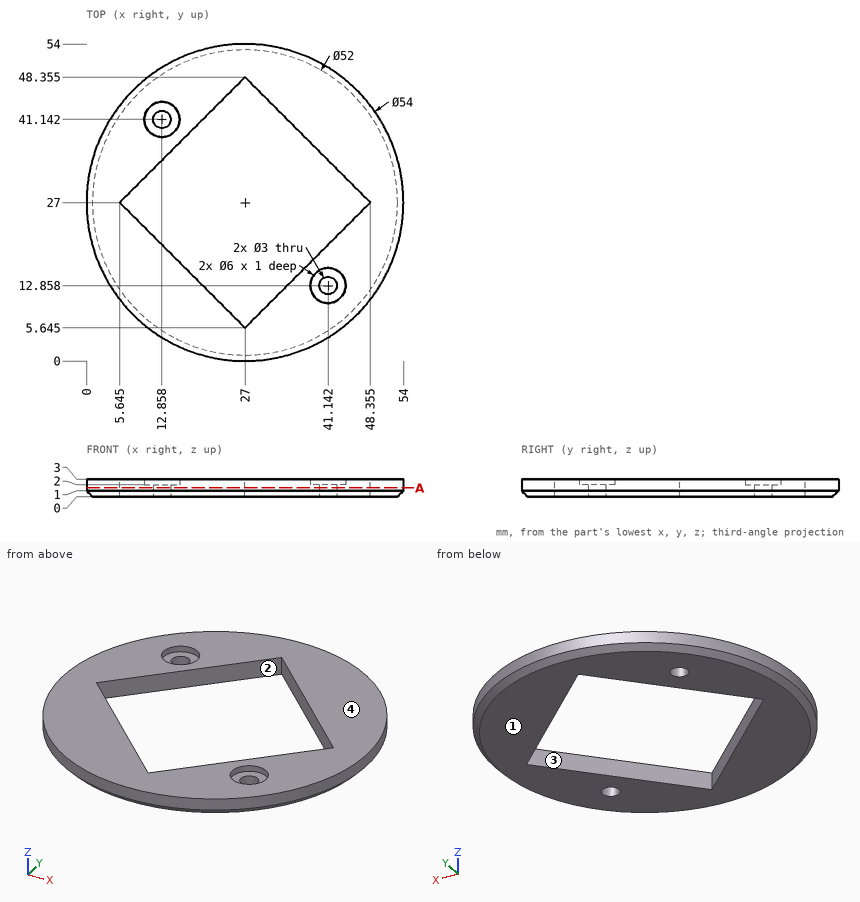
Input: dimensioned drawing with shaded views. Units: mm. Origin: part minimum x, y, z. A direction names the side the tool comes from. Round coordinates to 2 decimals unless told otherwise and drop trailing zeros. Loops run counter-clockwise (first coordinate to the right, second up) from the corner with the lowest first, then second, coordinate; pieces in that order, holes last. Notation, with made-up numbers: (-24.75, 44.25) -> (2.25, 44.25) arc R22 ccw to (2.25, 52.25) -> close; hole circle Ø7 at (-23, -28). An arc over 180 degrees is marked (long way). Use one line per item in the form item = value. Start each with the question number.
1) Section A-A on z = 1.5. Output: boundary loops of the cut face in (x, y) (1 decimal), then the cut area to 3 significant figures.
2) Access query for the marked faces 1 and 2. Directions: +Z, -Z, +X, -X, +Y, -Y. A direction counts if a zero-diameter tool reaches every point of the face in a straight line with its end or side. Return the directions, or none.
3) First-contact query: P1, Ø5, axis at x = 12.86, y = 41.14, coming from the +Z side; P2, Ø2.5, axis at x = 41.14, y = 12.86, coming from the +Z side; P3, Ø1.5, axis at x = 27, z = 1, coming from the -Y side. Flat tips, straight axial feed; report the tip coordinate or a pass-through.
4) Draft query along X for the marked faces 3 and 4. Return one class per face: released by +X, released by -X, zero draft, split by the parting line, or undercut.
5) Line query: L1, parallel to Y at x = 21, z = 2.6 (1 decimal); L2, parallel to Y at x = 38.5, z = 2.4 (1 decimal); L3, parallel to X at y = 22, z = 1.1 (1 decimal). Output: solid intervals per line, ascending.
Response:
q1.outline = circle Ø54 at (27, 27); hole (5.6, 27) -> (27, 5.6) -> (48.4, 27) -> (27, 48.4) -> close; hole circle Ø3 at (12.9, 41.1); hole circle Ø3 at (41.1, 12.9)
q1.area = 1,360 mm^2
q2.face_1 = -Z, +X, -X, +Y, -Y
q2.face_2 = +Z, -Z
q3.P1 = 2
q3.P2 = through
q3.P3 = 0
q4.face_3 = undercut
q4.face_4 = zero draft
q5.L1 = 0.7 to 11.6, 42.4 to 53.3
q5.L2 = 2.6 to 11.4, 14.3 to 17.1, 36.9 to 51.4
q5.L3 = 0.5 to 10.6, 43.4 to 53.5
